Here's how the part is built. I have some questions about the finished solid (model axes, mm). Round coordinates to 2 decimals unless told otherwise and drop trailing zeros. Write each loop counter-clockwise with the first axis right and the second up, starting at its lowest first coordinate (ties: lowest second). Pieces come first, ordered by that corner, then holes. Notation, with made-up numbers: (56, -24) - (106, -24) arc R23 cw to (106, -9) - close; hole circle Ø10 at (45, 73). An arc over 180 degrees is marked (long way). One line per item, written item: value. Start each with the question number.
Item 1: If I drill on line 1 (Z direction, x = -1.35, y = 50); line 2 (Y direction, x = 0.35, z = -35); line 3 (Y direction, x = -1.2, z = -76), over which ranges is the centre line in solid material (lowest first)?
Item 2: Imagine slicing it at C-C, the plane z = -67. Please give me the cut outline in (x, y).
Item 3: Imagine slicing it at B-B, the plane x = 1.05. Please give me the cut outline in (y, z), then the cut area to 3 significant figures.
Item 4: For P1, Ø1.5, axis at x = 0, z = -16.5, coming from the +Y side; P2, Ø1.5, axis at x = -0.5, y = 47, coming from the -Z side; P3, Ø1.5, axis at x = 0, z = 45.5, coming from the -Y side; P4, Ø7, axis at y = 255, z = 77, coming from the +X side, each with a flat end and sliding along its axis, tell me the tip position at first contact or that it passes through.
Item 5: Imagine slicing it at D-D, the plane y = 170. Please give me the cut outline in (x, z).
Item 6: Imagine slicing it at A-A, the plane y = 255. Please give me the cut outline in (x, z), then the cut area to 3 significant figures.
```python
from build123d import *

# Parameters (mm, degrees)
SKETCH_1_R             = 4
EXTRUDE_1_DEPTH        = 1.5
CUT_EXTRUDE_1_DEPTH    = 318.767533759
HOLE_WIZARD_M4_1_D     = 4.5
HOLE_WIZARD_M4_1_DEPTH = 4
HOLE_WIZARD_M4_1_TIP   = 1.351936393
SKETCH_5_W             = 30
SKETCH_5_H             = 60
CUT_EXTRUDE_2_DEPTH    = 318.767533759


with BuildPart() as part:
    # 草图1 → 凸台-拉伸1 (new, symmetric)
    with BuildSketch(Plane(origin=(0, 0, 0), x_dir=(0, 0, -1), z_dir=(1, 0, 0))):
        with BuildLine():
            Line((-27.769667841, 191.317400645), (-97.269946411, 251.221762497))
            Line((-97.269946411, 251.221762497), (-77.683571852, 273.9456251))
            Line((-77.683571852, 273.9456251), (-20.204886802, 224.403033058))
            ThreePointArc((-20.204886802, 224.403033058), (4.166491279, 210.007475855), (32.025445357, 205))
            Line((32.025445357, 205), (161, 205))
            Line((161, 205), (161, 0))
            Line((161, 0), (0, 0))
            Line((0, 0), (0, 130.720433703))
            ThreePointArc((0, 130.720433703), (-7.273022293, 164.048900719), (-27.769667841, 191.317400645))
        make_face()
        with Locations((-77, 255)):
            Circle(SKETCH_1_R, mode=Mode.SUBTRACT)
    extrude(amount=EXTRUDE_1_DEPTH, both=True)

    # 草图2 → 切除-拉伸1 (cut, through all)
    with BuildSketch(Plane(origin=(1.5, 0, 0), x_dir=(0, 0, -1), z_dir=(1, 0, 0))):
        with BuildLine():
            Line((37, 0), (107, 0))
            Line((107, 0), (107, 65))
            ThreePointArc((107, 65), (104.071067812, 72.071067812), (97, 75))
            Line((97, 75), (47, 75))
            ThreePointArc((47, 75), (39.928932188, 72.071067812), (37, 65))
            Line((37, 65), (37, 0))
        make_face()
    extrude(amount=-CUT_EXTRUDE_1_DEPTH, mode=Mode.SUBTRACT)

    # M4 间隙孔1
    with Locations(Plane(origin=(1.5, 0, 0), x_dir=(0, 0, -1), z_dir=(1, 0, 0))):
        with Locations((34.69, 157.500209205), (24, 102.53), (153.464916317, 134.40217349), (142.774916317, 79.431964286)):
            Hole(HOLE_WIZARD_M4_1_D / 2, depth=HOLE_WIZARD_M4_1_DEPTH)
            with Locations((0, 0, -(HOLE_WIZARD_M4_1_DEPTH + HOLE_WIZARD_M4_1_TIP / 2))):  # 118° drill point
                Cone(0, HOLE_WIZARD_M4_1_D / 2, HOLE_WIZARD_M4_1_TIP, mode=Mode.SUBTRACT)

    # 草图5 → 切除-拉伸2 (cut, through all)
    with BuildSketch(Plane(origin=(1.5, 0, 0), x_dir=(0, 0, -1), z_dir=(1, 0, 0))):
        with Locations((146, 30)):
            Rectangle(SKETCH_5_W, SKETCH_5_H)
    extrude(amount=-CUT_EXTRUDE_2_DEPTH, mode=Mode.SUBTRACT)


solid = part.part
```
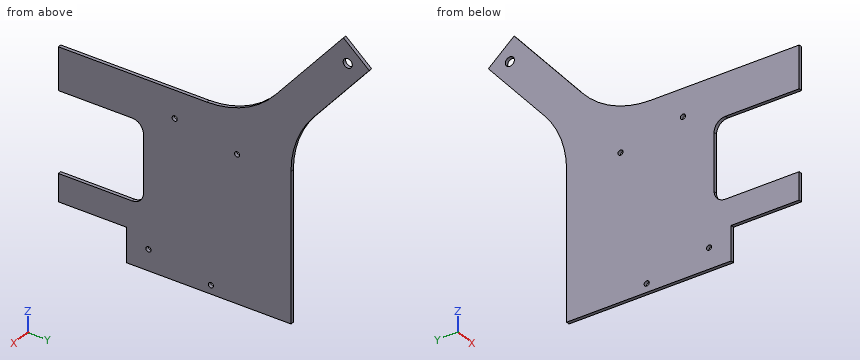
Values follow:
1. line 1: z = -131 to -107, -37 to 0
1. line 2: y = 0 to 155.27, 159.73 to 205
1. line 3: y = 75 to 205
2. outline: (-1.5, 75) - (1.5, 75) - (1.5, 205) - (-1.5, 205) - close
3. outline: (0, -131) - (60, -131) - (60, -161) - (205, -161) - (205, -32.03) arc R80 cw to (224.4, 20.2) - (273.95, 77.68) - (251.22, 97.27) - (191.32, 27.77) arc R80 cw to (130.72, 0) - (0, 0) - (0, -37) - (65, -37) arc R10 cw to (75, -47) - (75, -97) arc R10 cw to (65, -107) - (0, -107) - close; hole circle Ø4.5 at (79.43, -142.77); hole circle Ø4.5 at (102.53, -24); hole circle Ø4.5 at (134.4, -153.46); hole circle Ø4.5 at (157.5, -34.69); hole circle Ø8 at (255, 77)
3. area: 29,600 mm^2
4. P1: stops at y = 206.67
4. P2: stops at z = -131
4. P3: stops at y = 205.95
4. P4: passes through
5. outline: (-1.5, -161) - (1.5, -161) - (1.5, 10.31) - (-1.5, 10.31) - close
6. outline: (-1.5, 55.7) - (1.5, 55.7) - (1.5, 73) - (-1.5, 73) - close; (-1.5, 81) - (1.5, 81) - (1.5, 94.01) - (-1.5, 94.01) - close
6. area: 90.9 mm^2
